from build123d import *

# Parameters (mm, degrees)
BOSS_EXTRUDE1_DEPTH        = 3.175
F_1_8_0_1250_DOWEL_HOLE2_D = 3.175
SKETCH7_W                  = 3.175
SKETCH7_H                  = 19.05
BOSS_EXTRUDE2_DEPTH        = 15.875
F_8_CLEARANCE_HOLE1_D      = 4.4958


with BuildPart() as part:
    # Sketch1 → Boss-Extrude1 (new body)
    with BuildSketch(Plane.XY):
        Polygon((0, 0), (-22.225, 0), (-22.225, -6.35), (-6.35, -19.05), (0, -19.05), align=None)
    extrude(amount=BOSS_EXTRUDE1_DEPTH)

    # 1/8 (0.1250) Dowel Hole2 (through all)
    with Locations(Plane.XY.offset(3.175)):
        with Locations((-11.1125, -3.175)):
            Hole(F_1_8_0_1250_DOWEL_HOLE2_D / 2)

    # Sketch7 → Boss-Extrude2 (add)
    with BuildSketch(Plane.XY.offset(3.175)):
        with Locations((-1.5875, -9.525)):
            Rectangle(SKETCH7_W, SKETCH7_H)
    extrude(amount=-BOSS_EXTRUDE2_DEPTH)

    # #8 Clearance Hole1 (through all)
    with Locations(Plane.ZY.offset(3.175)):
        with Locations((-6.35, -15.875), (-6.35, -3.175)):
            Hole(F_8_CLEARANCE_HOLE1_D / 2)


solid = part.part
Can you work these out from the model? Positions are in its coordinate system, mm. A direction names the side the tool comes from. Give positions to 0.01 mm unless a question says otherwise; leave off trailing zeros. Loops run counter-clockwise (first coordinate to the right, second up) from the corner with the lowest first, then second, coordinate; pieces in that order, holes last. Notation, with made-up numbers: (66, -4.75) -> (84, -4.75) arc R23 cw to (84, 14.25) -> close; hole circle Ø4 at (-24.75, 89). An arc over 180 degrees is marked (long way). Use one line per item in the form item = value.
1) If we section it at D-D (x = -2.25): Please give me the cut outline in (y, z) (3 decimals).
Answers:
outline = (-19.05, -12.7) -> (0, -12.7) -> (0, 3.175) -> (-19.05, 3.175) -> close; hole circle Ø4.496 at (-15.875, -6.35); hole circle Ø4.496 at (-3.175, -6.35)
2) Will these pins go through, and if not, where does the flat tip stop? pin 1 (2 mm diameter, centred on x = -15.5, z = 1, fed in from -Y); pin 2 (5 mm diameter, centred on y = -3.175, z = -6.35, fed in from -X) (3 decimals).
Answers:
pin_1 = -12.53
pin_2 = -3.175
3) If we section it at A-A (z = -6.35): Please give me the cut outline in (x, y) (3 decimals).
Answers:
outline = (-3.175, -19.05) -> (0, -19.05) -> (0, -18.123) -> (-3.175, -18.123) -> close; (-3.175, -13.627) -> (0, -13.627) -> (0, -5.423) -> (-3.175, -5.423) -> close; (-3.175, -0.927) -> (0, -0.927) -> (0, 0) -> (-3.175, 0) -> close
4) For faces 5 (the face through (-11, -7, 0)), 6 (the face through (-1.57, -18.07, -5.86)), which set-ups out of +Z, -Z, +X, -X, +Y, -Y let a thin tool reach every point of the face, with its end or its side?
Answers:
face_5 = -Z, -X, +Y, -Y
face_6 = +X, -X
5) We'd pull the mould along Y, two halves only. Please class faces 1 (the face through (-6.9, 0, 0.5)), 2 (the face through (-22.225, -3, 2)), 3 (the face through (-12.58, -3.78, 1.57)), 4 (the face through (-14.4, -12.61, 1.57)): released by +Y, released by -Y, zero draft, split by the parting line, or undercut.
Answers:
face_1 = released by +Y
face_2 = zero draft
face_3 = undercut
face_4 = released by -Y
6) If we section it at B-B (y = -14.75): Please give me the cut outline in (x, z) (3 decimals), plus the area to 3 significant figures.
Answers:
outline = (-11.725, 0) -> (-3.175, 0) -> (-3.175, -4.404) -> (0, -4.404) -> (0, 3.175) -> (-11.725, 3.175) -> close; (-3.175, -12.7) -> (0, -12.7) -> (0, -8.296) -> (-3.175, -8.296) -> close
area = 65.2 mm²
7) I need wall thicknesses on line 1 along Y through (x, z) = (-2.25, -6.35); line 2 along Y through (x, z) = (-1, -8); line 3 along Z through (x, y) = (-19, -3.25) (3 decimals). Which ranges of each line are inside material? Lowest first, please.
Answers:
line_1 = -19.05 to -18.12, -13.63 to -5.42, -0.93 to 0
line_2 = -19.05 to -17.4, -14.35 to -4.7, -1.65 to 0
line_3 = 0 to 3.175
